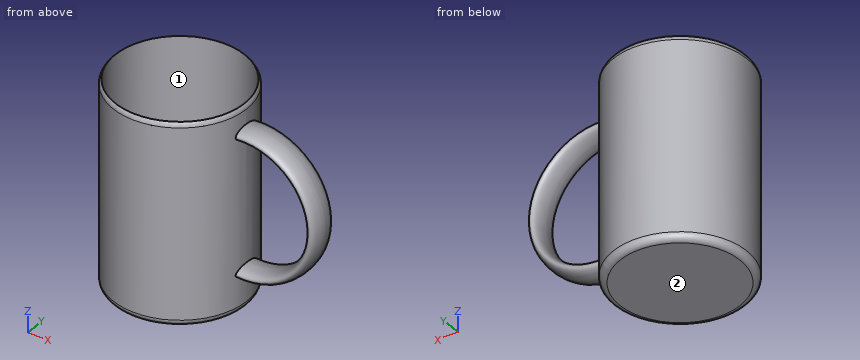
from build123d import *

# Parameters (mm, degrees)
F0_R     = 50.8
F0_R_2   = 49.2125
F1_DEPTH = 152.4
F2_DEPTH = 3.175
F7_R     = 5.08


# Not quite as in the source:
# - a fillet or chamfer that OpenCascade refuses, or shapes differently, is made with other operations: its cross-section is extruded or revolved along the edge and cut away or added


with BuildPart() as f1:
    # F0 (on Top) → F1 (new body)
    with BuildSketch(Plane.XY):
        with Locations((-50.7995303897, 0.2184311975)):
            Circle(F0_R)
        with Locations((-50.7995303897, 0.2184311975)):
            Circle(F0_R_2, mode=Mode.SUBTRACT)
    extrude(amount=F1_DEPTH)

    # F0 (on Top) → F2 (join)
    with BuildSketch(Plane.XY):
        with Locations((-50.7995303897, 0.2184311975)):
            Circle(F0_R_2)
    extrude(amount=F2_DEPTH)

    # F5: sweep along a path in F4
    with BuildLine(Plane.XZ) as f5_path:
        ThreePointArc((0, 31.0402940959), (56.0160848718, 82.0873966441), (0, 133.1344991922))
    # F3 (on Right) → F5 (sweep)
    with BuildSketch(Plane.YZ):
        with BuildLine():
            add(Edge.make_bspline(
                [(11.1326146871, 133.4060281515), (11.1326146871, 141.0279565911), (-5.5663073435, 137.2169923713), (-22.2652293742, 133.4060281515), (-5.5663073435, 129.5950639317), (11.1326146871, 125.7840997119), (11.1326146871, 133.4060281515)],
                knots=[0, 0, 0, 2.0943951024, 2.0943951024, 4.1887902048, 4.1887902048, 6.2831853072, 6.2831853072, 6.2831853072], degree=2, weights=[1, 0.5, 1, 0.5, 1, 0.5, 1]))
        make_face()
    sweep(path=f5_path.line)

    # F6: fillet of radius 5.08 on 1 edges, made by hand

    # F6_s1 → F6_t2 (revolve, cut)
    with BuildSketch(Plane.XZ.offset(-0.2184311975)):
        with BuildLine():
            ThreePointArc((0.0008696103, 148.7105678213), (-0.412881514, 150.7189630856), (-1.5867553659, 152.4002904513))
            Line((-1.5867553659, 152.4002904513), (-1.237381295, 152.7692627143))
            ThreePointArc((-1.237381295, 152.7692627143), (-0.7931428778, 152.9081365685), (0.0004696103, 152.9081365685))
            Line((0.0004696103, 152.9081365685), (0.5086061789, 152.4))
            ThreePointArc((0.5086061789, 152.4), (0.5086061789, 150.5552839107), (0.5090061789, 148.7105678213))
            Line((0.5090061789, 148.7105678213), (0.0008696103, 148.7105678213))
        make_face()
    revolve(axis=Axis((-50.7995303897, 0.2184311975, 152.4), (0, 0, 1)), mode=Mode.SUBTRACT)

    # F7
    f7_edges = [f1.edges().sort_by_distance(p)[0] for p in [
        (-101.59953, 0.218431, 0),
    ]]
    fillet(f7_edges, radius=F7_R)


solid = f1.part
Geometry: final body of the model. Coordinates: model frame, mm. Face numbers are marked on the shaded views. Give positions to 0.01 mm unless a question says otherwise; leave off trailing zeros. Order: outer loops, then holes, each group sorted by start corner. A loop starts at its lowest first (then second) coordinate and runs counter-clockwise, first axis right, second up. Notation, with made-up numbers: (21, 61.5) - (54, 61.5) arc R17 cw to (54, 92.5) - close; hole circle Ø11 at (39, 17.5). An arc over 180 degrees is marked (long way). Use CSV: the item, a comma, the result in double quotes.
1. Material intervals for line 1 along Y through (x, z) = (-50, 7); line 2 along Z through (x, y) = (-23, -32.5) (3 decimals); line 3 along Y through (x, z) = (-13, 123), sorted ascending. Write a range as from..to.
Answers below:
line 1,"-50.58..-48.99, 49.42..51.01"
line 2,"0..3.175"
line 3,"-33.72..-31.29, 31.73..34.16"
2. Section query B-B (z = 12). Output: boundary loops of the cut face in (x, y) (1 decimal).
Answers below:
outline,"circle Ø101.6 at (-50.8, 0.2); hole circle Ø98.4 at (-50.8, 0.2)"
3. Contact query for flat-ended pins moving along their axis: pin 1 (6 mm diameter, centred on y = -4.5, z = 46.5, fed in from +X); pin 2 (4.5 mm diameter, centred on y = -3.5, z = 132.5, fed in from -X); pin 3 (6 mm diameter, centred on x = -27.5, z = 89, fed in from +Y). Output: stop coordinate, or through.
Answers below:
pin 1,"x = 49.81"
pin 2,"x = -101.58"
pin 3,"y = 46.79"
4. Section query A-A (z = 69.5). Give the number of separate pieces and of enclosed holes in the cut face, plus the area to 3 significant figures.
Answers below:
separate pieces,"2"
enclosed holes,"1"
area,"657 mm2"
5. Mould query, pull axis Y, two halves, no side actions, for the marked faces 1 and 2. Classes: +Y half, -Y half, draft (parallel to the pull), parting line (faces both ways), or undercut.
Answers below:
face 1,"undercut"
face 2,"draft"
